Answer from the drawing. Dimensions are ordinates in mm from the lowest x, y and z of the part. A direction names the side the tool comes from. Coordinates: 2 decimals unless noted, no trailing zeros. Order: outer loops, then holes, each group sorted by start corner. A loop starts at its lowest first (then second) coordinate and runs counter-clockwise, first axis right, second up. Notation, with made-up numbers: (32, 21) - (83, 21) arc R8 ccw to (83, 26) - close; hole circle Ø10 at (77, -31.75). An arc over 180 degrees is marked (long way). Answer as a JSON object with one key per item and string values. Group by question number.
1) Section B-B (y = 25) is taken. Give the vertices of the cut face in (x, z).
2) The mould has two halves that part along Y. Classify the marked faces 1, 2, 3 and 4: released by +Y, released by -Y, zero draft, split by the parting line, or undercut.
3) Find the intervals of material crossed by line 1 along X through (y, z) = (18, 41.5); line 2 along Y through (x, z) = (36, 44.5); line 3 along X through (y, z) = (1.15, 30), in increasing order.
4) Section D-D (z = 11.5) is taken. Give the vertices of the cut face in (x, y).
5) Section A-A (x = 21) is taken. Give the vertices of the cut face in (y, z), plus the area to 3 significant figures.
6) Section C-C (x = 30) is taken. Give the vertices of the cut face in (y, z), plus the area to 4 significant figures.
7) A tool of negligible diameter and unlimited length cuts with its end or side. For the marked faces 5 and 6, from which of +Z, -Z, +X, -X, +Y, -Y can it reach the whole face along a straight path? Write none if from no direction.
8) Each of these flat-tipped pins is pushed along its axis until it touches: P1, Ø12, axis at x = 51, y = 13.5, coming from the +Z side; P2, Ø5, axis at x = 16, y = 4, coming from the -Z side; P3, Ø1.5, axis at x = 26.5, z = 9.5, coming from the +Y side. Where does it stop, or does it pass through?
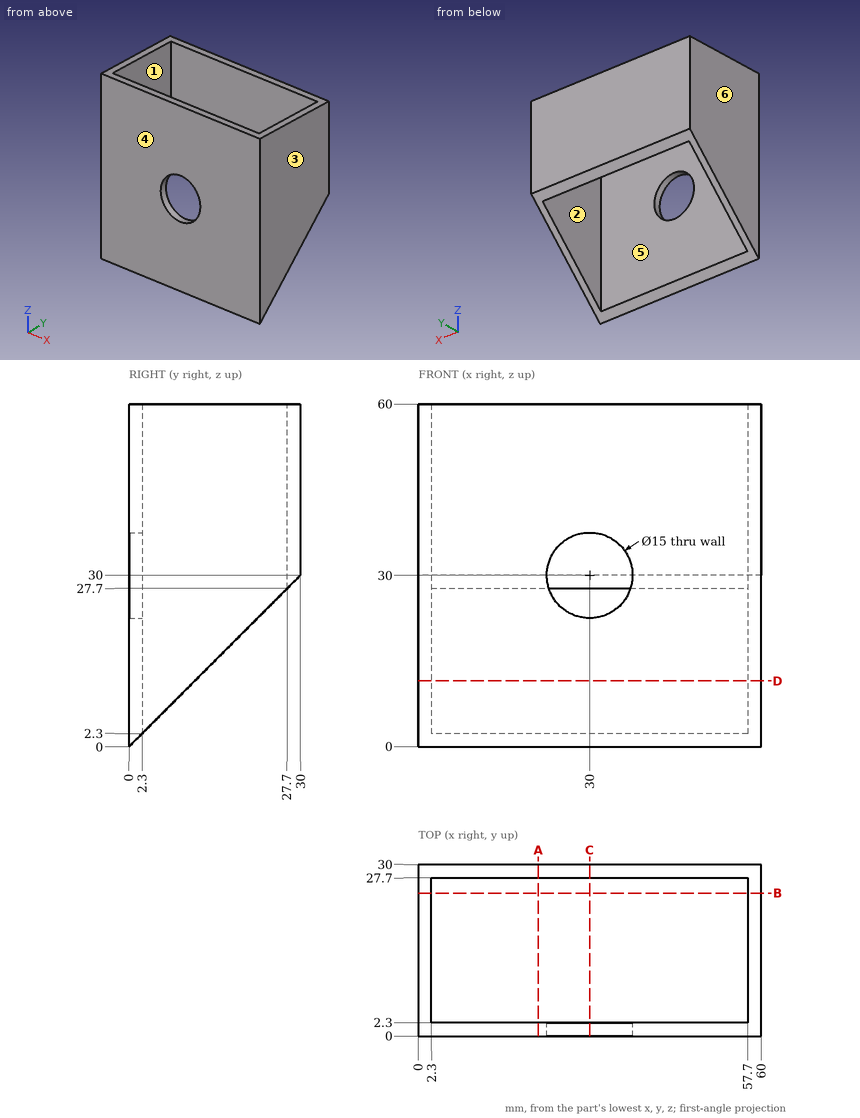
Report:
{
 "1": {"outline": "(0, 25) - (2.3, 25) - (2.3, 60) - (0, 60) - close; (57.7, 25) - (60, 25) - (60, 60) - (57.7, 60) - close"},
 "2": {"face 1": "undercut", "face 2": "undercut", "face 3": "zero draft", "face 4": "released by -Y"},
 "3": {"line 1": "x = 0 to 2.3, 57.7 to 60", "line 2": "y = 0 to 2.3, 27.7 to 30", "line 3": "x = 0 to 22.5, 37.5 to 60"},
 "4": {"outline": "(0, 0) - (60, 0) - (60, 11.5) - (57.7, 11.5) - (57.7, 2.3) - (2.3, 2.3) - (2.3, 11.5) - (0, 11.5) - close"},
 "5": {"outline": "(0, 0) - (2.3, 2.3) - (2.3, 60) - (0, 60) - close; (27.7, 27.7) - (30, 30) - (30, 60) - (27.7, 60) - close", "area": "207 mm²"},
 "6": {"outline": "(0, 0) - (2.3, 2.3) - (2.3, 22.5) - (0, 22.5) - close; (0, 37.5) - (2.3, 37.5) - (2.3, 60) - (0, 60) - close; (27.7, 27.7) - (30, 30) - (30, 60) - (27.7, 60) - close", "area": "172.5 mm²"},
 "7": {"face 5": "+Z, -Z", "face 6": "+Z, -Z, -X, +Y, -Y"},
 "8": {"P1": "passes through", "P2": "stops at z = 1.5", "P3": "stops at y = 2.3"}
}
